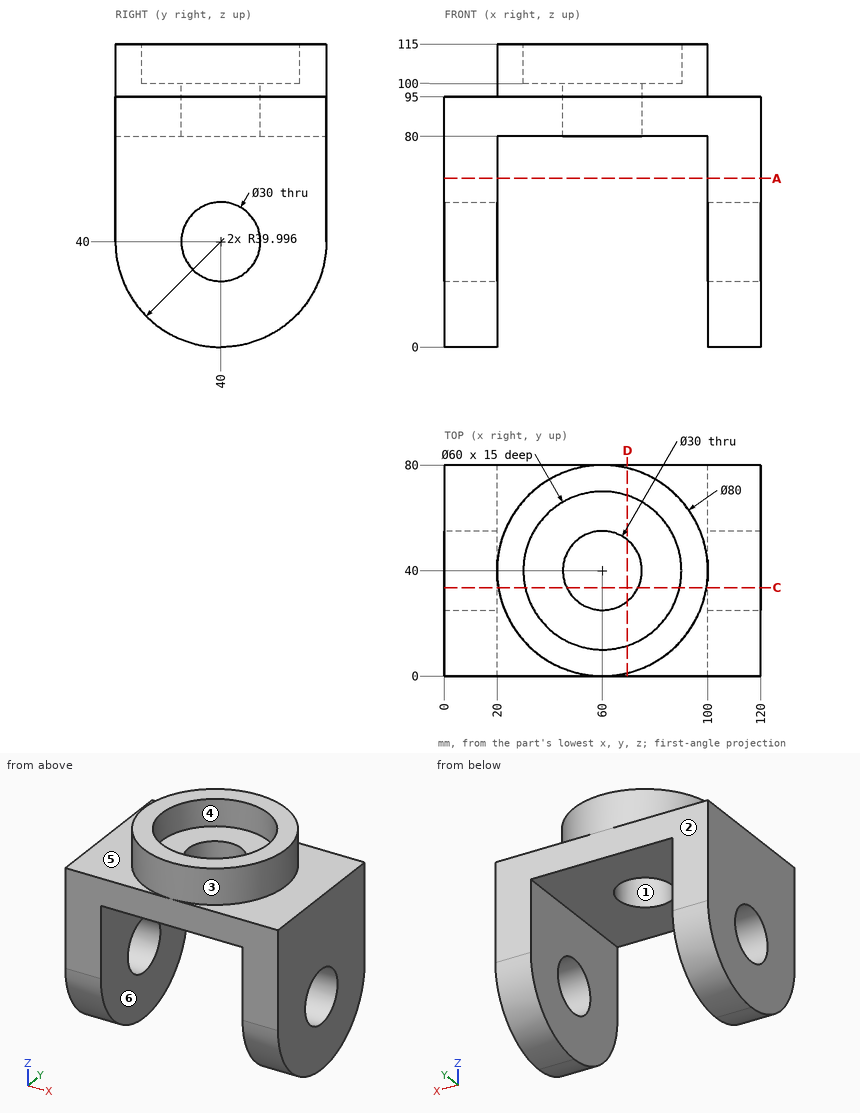
The drawing under review shows one solid part. Ordinate dimensions are in mm from its lowest x, y, z. A direction names the side the tool comes from. Give positions to 0.01 mm unless a question says otherwise; leave off trailing zeros. Order: outer loops, then holes, each group sorted by start corner. A loop starts at its lowest first (then second) coordinate and runs counter-clockwise, first axis right, second up. Notation, with made-up numbers: (40.5, 44.25) -> (66.5, 44.25) arc R20 ccw to (66.5, 60.25) -> close; hole circle Ø4 at (14.5, 48). An arc over 180 degrees is marked (long way). Write item = value, one per line. Start each with the question number.
(1) We need section C-C on y = 33.5. Write out the cut boundary in (x, z).
(2) For the marked faces 4, 5 and 6, list the 3-axis set-ups (+Z, -Z, +X, -X, +Y, -Y) from which the entire face can be reached by the end or side of a thin tool; tool diameter is ignored.
(3) We need section A-A on z = 64. Write out the cut boundary in (x, y), plus the area to 3 significant figures.
(4) We need section D-D on x = 69.5. Write out the cut boundary in (y, z).
(5) To check wall thickness, follow line 1 along X through (y, z) = (66, 62); line 2 along Y through (x, z) = (60, 105.5); line 3 along Z through (x, y) = (109, 40). State the ranges of each line that lie inside material, in increasing order.
(6) For pin 1 (3 mm diameter, centred on x = 71, y = 19.5, fed in from +Z); pin 2 (18 mm diameter, centred on y = 40, z = 40, fed in from +X); pin 3 (2 mm diameter, centred on x = 19, y = 54, fed in from +Z), all flat-tipped, find the tip position at first contact; note any pin that passes through.
(7) Mouldability with a two-part tool opening along X and no side actions: class the marked faces 1, 2 and 3 as +X half, -X half, draft (parallel to the pull), parting line (faces both ways), or undercut.
Numbers:
q1.outline = (0, 0.53) -> (20, 0.53) -> (20, 26.48) -> (0, 26.48) -> close; (0, 53.52) -> (20, 53.52) -> (20, 80) -> (46.48, 80) -> (46.48, 100) -> (30.71, 100) -> (30.71, 115) -> (20.53, 115) -> (20.53, 95) -> (0, 95) -> close; (73.52, 80) -> (100, 80) -> (100, 53.52) -> (120, 53.52) -> (120, 95) -> (99.47, 95) -> (99.47, 115) -> (89.29, 115) -> (89.29, 100) -> (73.52, 100) -> close; (100, 0.53) -> (120, 0.53) -> (120, 26.48) -> (100, 26.48) -> close
q2.face_4 = +Z
q2.face_5 = +Z, -X
q2.face_6 = -Z, +Y, -Y
q3.outline = (0, 0) -> (20, 0) -> (20, 80) -> (0, 80) -> close; (100, 0) -> (120, 0) -> (120, 80) -> (100, 80) -> close
q3.area = 3,200 mm^2
q4.outline = (0, 80) -> (28.39, 80) -> (28.39, 100) -> (11.54, 100) -> (11.54, 115) -> (1.14, 115) -> (1.14, 95) -> (0, 95) -> close; (51.61, 80) -> (80, 80) -> (80, 95) -> (78.86, 95) -> (78.86, 115) -> (68.46, 115) -> (68.46, 100) -> (51.61, 100) -> close
q5.line_1 = 0 to 20, 100 to 120
q5.line_2 = 0 to 10, 70 to 80
q5.line_3 = 0 to 25, 55 to 95
q6.pin_1 = 100
q6.pin_2 = through
q6.pin_3 = 95
q7.face_1 = undercut
q7.face_2 = draft
q7.face_3 = parting line
